from build123d import *

# Parameters (mm, degrees)
SKETCH1_W               = 50.8
SKETCH1_H               = 50.8
BOSS_EXTRUDE1_DEPTH     = 25.4
SKETCH2_R               = 4.7625
CUT_EXTRUDE1_DEPTH      = 63.217039467
F_1_4_CLEARANCE_HOLE1_D = 6.7564
SKETCH6_R               = 3.175
CUT_EXTRUDE2_DEPTH      = 63.217039467
F_8_CLEARANCE_HOLE1_D   = 4.4958


with BuildPart() as part:
    # Sketch1 → Boss-Extrude1 (new body)
    with BuildSketch(Plane(origin=(0, 0, 0), x_dir=(1, 0, 0), z_dir=(0, 1, 0))):
        Rectangle(SKETCH1_W, SKETCH1_H)
    extrude(amount=BOSS_EXTRUDE1_DEPTH)

    # Sketch2 → Cut-Extrude1 (cut, through all)
    with BuildSketch(Plane.XY.offset(25.4)):
        with Locations((-9.525, 25.4)):
            Circle(SKETCH2_R)
        with Locations((9.525, 25.4)):
            Circle(SKETCH2_R)
    extrude(amount=-CUT_EXTRUDE1_DEPTH, mode=Mode.SUBTRACT)

    # 1/4 Clearance Hole1 (through all)
    with Locations(Plane(origin=(0, 25.4, 0), x_dir=(1, 0, 0), z_dir=(0, 1, 0))):
        with Locations((-19.05, 19.05), (-19.05, -19.05), (19.05, -19.05), (19.05, 19.05)):
            Hole(F_1_4_CLEARANCE_HOLE1_D / 2)

    # Sketch6 → Cut-Extrude2 (cut, through all)
    with BuildSketch(Plane.XY.offset(25.4)):
        with Locations((-9.525, 12.7)):
            Circle(SKETCH6_R)
        with Locations((9.525, 12.7)):
            Circle(SKETCH6_R)
    extrude(amount=-CUT_EXTRUDE2_DEPTH, mode=Mode.SUBTRACT)

    # #8 Clearance Hole1 (through all)
    with Locations(Plane(origin=(0, 25.4, 0), x_dir=(1, 0, 0), z_dir=(0, 1, 0))):
        with Locations((0, 12.7), (0, -12.7)):
            Hole(F_8_CLEARANCE_HOLE1_D / 2)


solid = part.part
Check sheet for the modelled part. Datum: model origin and axes. Units: mm. Round coordinates to 2 decimals unless told otherwise and drop trailing zeros. Write each loop counter-clockwise with the first axis right and the second up, starting at its lowest first coordinate (ties: lowest second). Pieces come first, ordered by that corner, then holes. Notation, with made-up numbers: (27.5, -37.75) -> (51.5, -37.75) arc R8 cw to (51.5, -26.75) -> close; hole circle Ø6 at (10.25, 79.25). An arc over 180 degrees is marked (long way). Answer as CSV lines item,"result". Start each with the question number.
1) Section check B-B on x = 19.05. Enter the section's corners in (y, z), and give its area (3 significant figures).
2) Go/stop test with a flat-tipped pin: P1, Ø2.5, axis at x = 0, z = 12.7, coming from the -Y side. Record where the tip stops, or that it passes through.
3) Release check for a two-part mould opening along Y. For faces 1 (the flat face through (0, 25.4, 0)), 2 (the cylindrical face through (-12.045, 10.768, 0.356)), 3 (the flat face through (0, 13, 25.4)) record: pulls with the +Y half, pulls with the -Y half, needs draft (parallel to the pull), parting line crosses it, or undercut.
4) Material ranges on line 1 (Z direction, x = 0, y = 16); line 2 (X direction, y = 20.25, z = -19.05), recorded low to high. Write a range as from..to.
5) Section check A-A on z = -12.7. State how many separate pieces and enclosed holes the cut face has, and give its area (3 significant figures).
Found:
1,outline,"(0, -25.4) -> (25.4, -25.4) -> (25.4, -22.43) -> (0, -22.43) -> close; (0, -15.67) -> (25.4, -15.67) -> (25.4, 15.67) -> (0, 15.67) -> close; (0, 22.43) -> (25.4, 22.43) -> (25.4, 25.4) -> (0, 25.4) -> close"
1,area,"947 mm^2"
2,P1,"passes through"
3,face 1,"pulls with the +Y half"
3,face 2,"undercut"
3,face 3,"needs draft"
4,line 1,"z = -25.4..-14.95, -10.45..10.45, 14.95..25.4"
4,line 2,"x = -25.4..-22.43, -15.67..15.67, 22.43..25.4"
5,separate pieces,"2"
5,enclosed holes,"2"
5,area,"1,040 mm^2"
